Design review of the part built by this model. Coordinates are the model's own, in mm. A direction names the side the tool comes from. Give positions to 0.01 mm unless a question says otherwise; leave off trailing zeros. Loops run counter-clockwise (first coordinate to the right, second up) from the corner with the lowest first, then second, coordinate; pieces in that order, holes last. Notation, with made-up numbers: M 71.25,80.5 L 97.25,80.5 A14 cw 97.25,88.5 Z; hole C 52,87.25 d5. An arc over 180 degrees is marked long. Use a Markdown table: item, result. Add a question column.
(1) For probe 1 along Z at (x, y) = (63, 20); probe 2 along X at (y, z) = (20.5, 14); probe 3 along Z at (x, y) = (24, 15), list the stretches that pass through material, from the lowest coordinate up.
(2) Add section B-B, the plane x = -1.5. Give the boundary of the cut face in (y, z).
(3) Add section D-D, the plane x = 38.5. Give the boundary of the cut face in (y, z), then the cut area to 3 significant figures.
(4) Add section C-C, the plane z = 37. Give the boundary of the cut face in (x, y).
(5) Insertion check: pin 1 Ø24 at (x, y) = (53, 21) entering from -Z; pin 2 Ø15 at (x, z) = (2, 50) entering from -Y; pin 3 Ø12 at (x, y) = (11.5, 7.5) entering from -Z; pin 4 Ø5 at (x, y) = (-24, 26) entering from -Z. Each pin has a flat end and moves straight along its axis. Give the tip position at first contact, or say it passes through.
(6) Add section A-A, the plane z = 11. Give the boundary of the cut face in (x, y), then the cut area to 3 significant figures.
(7) Draft analysis for pull direction Z (two halves, no side actions). For faces 5 (the face through (23, 20, 18)), 6 (the face through (-50, 20, -15)), 7 (the face through (0, 7, -49)), state which applies: pulls with the +Z half, pulls with the -Z half, needs draft (parallel to the pull), parting line crosses it, or undercut.
(8) For faces 1 (the face through (18, 20, 23)), 2 (the face through (0, 33, 49)), 3 (the face through (-50, 20, 15)), 4 (the face through (49, 7, 0)), list the 3-axis set-ups (+Z, -Z, +X, -X, +Y, -Y) from which the entire face can be reached by the end or side of a thin tool; tool diameter is ignored.
```python
from build123d import *

# Parameters (mm, degrees)
CROQUIS1_W     = 40
CROQUIS1_H     = 50
CROQUIS1_H_2   = 40
CROQUIS1_W_2   = 50
EXTRUIR1_DEPTH = 40
CROQUIS2_W     = 40
CROQUIS2_H     = 40
CROQUIS2_W_2   = 30
CROQUIS2_H_2   = 30
EXTRUIR2_DEPTH = 40
CROQUIS3_W     = 40
CROQUIS3_H     = 40
CROQUIS3_W_2   = 30
CROQUIS3_H_2   = 30
EXTRUIR3_DEPTH = 40
CROQUIS5_W     = 40
CROQUIS5_H     = 40
CROQUIS5_W_2   = 30
CROQUIS5_H_2   = 30
EXTRUIR4_DEPTH = 40
CROQUIS6_W     = 40
CROQUIS6_H     = 40
CROQUIS6_W_2   = 30
CROQUIS6_H_2   = 30
EXTRUIR5_DEPTH = 40
VACIADO1_T     = -2


with BuildPart() as part:
    # Croquis1 → Extruir1 (new body)
    with BuildSketch(Plane(origin=(0, 0, 0), x_dir=(1, 0, 0), z_dir=(0, 1, 0))):
        with Locations((0, 45)):
            Rectangle(CROQUIS1_W, CROQUIS1_H)
        Rectangle(CROQUIS1_W, CROQUIS1_H_2)
        with Locations((45, 0)):
            Rectangle(CROQUIS1_W_2, CROQUIS1_H_2)
        with Locations((-45, 0)):
            Rectangle(CROQUIS1_W_2, CROQUIS1_H_2)
        with Locations((0, -45)):
            Rectangle(CROQUIS1_W, CROQUIS1_H)
    extrude(amount=EXTRUIR1_DEPTH)

    # Croquis2 → Extruir2 (cut)
    with BuildSketch(Plane(origin=(70, 0, 0), x_dir=(0, 0, -1), z_dir=(1, 0, 0))):
        with Locations((0, 20)):
            Rectangle(CROQUIS2_W, CROQUIS2_H)
        with Locations((0, 20)):
            Rectangle(CROQUIS2_W_2, CROQUIS2_H_2, mode=Mode.SUBTRACT)
    extrude(amount=-EXTRUIR2_DEPTH, mode=Mode.SUBTRACT)

    # Croquis3 → Extruir3 (cut)
    with BuildSketch(Plane(origin=(0, 0, -70), x_dir=(-1, 0, 0), z_dir=(0, 0, -1))):
        with Locations((0, 20)):
            Rectangle(CROQUIS3_W, CROQUIS3_H)
        with Locations((0, 20)):
            Rectangle(CROQUIS3_W_2, CROQUIS3_H_2, mode=Mode.SUBTRACT)
    extrude(amount=-EXTRUIR3_DEPTH, mode=Mode.SUBTRACT)

    # Croquis5 → Extruir4 (cut)
    with BuildSketch(Plane.ZY.offset(70)):
        with Locations((0, 20)):
            Rectangle(CROQUIS5_W, CROQUIS5_H)
        with Locations((0, 20)):
            Rectangle(CROQUIS5_W_2, CROQUIS5_H_2, mode=Mode.SUBTRACT)
    extrude(amount=-EXTRUIR4_DEPTH, mode=Mode.SUBTRACT)

    # Croquis6 → Extruir5 (cut)
    with BuildSketch(Plane.XY.offset(70)):
        with Locations((0, 20)):
            Rectangle(CROQUIS6_W, CROQUIS6_H)
        with Locations((0, 20)):
            Rectangle(CROQUIS6_W_2, CROQUIS6_H_2, mode=Mode.SUBTRACT)
    extrude(amount=-EXTRUIR5_DEPTH, mode=Mode.SUBTRACT)

    # Vaciado1
    vaciado1_openings = [part.faces().sort_by_distance(p)[0] for p in [
        (0, 20, 70),
        (70, 20, 0),
        (0, 20, -70),
        (-70, 20, 0),
    ]]
    offset(amount=VACIADO1_T, openings=vaciado1_openings, kind=Kind.INTERSECTION)


solid = part.part
```
Established:
| question | item | result |
|---|---|---|
| 1 | probe 1 | -15 to -13, 13 to 15 |
| 1 | probe 2 | -70 to -28, 28 to 70 |
| 1 | probe 3 | -20 to -18, 18 to 20 |
| 2 | outline | M 0,-30 L 5,-30 L 5,-70 L 7,-70 L 7,-28 L 2,-28 L 2,28 L 7,28 L 7,70 L 5,70 L 5,30 L 0,30 Z; M 33,-70 L 35,-70 L 35,-30 L 40,-30 L 40,30 L 35,30 L 35,70 L 33,70 L 33,28 L 38,28 L 38,-28 L 33,-28 Z |
| 3 | outline | M 5,-15 L 35,-15 L 35,15 L 5,15 Z; hole M 7,-13 L 33,-13 L 33,13 L 7,13 Z |
| 3 | area | 224 mm^2 |
| 4 | outline | M -15,5 L 15,5 L 15,35 L -15,35 Z; hole M -13,7 L 13,7 L 13,33 L -13,33 Z |
| 5 | pin 1 | z = -15 |
| 5 | pin 2 | y = 5 |
| 5 | pin 3 | z = -70 |
| 5 | pin 4 | z = -20 |
| 6 | outline | M -70,5 L -30,5 L -30,0 L 30,0 L 30,5 L 70,5 L 70,7 L 28,7 L 28,2 L -28,2 L -28,7 L -70,7 Z; M -70,33 L -28,33 L -28,38 L 28,38 L 28,33 L 70,33 L 70,35 L 30,35 L 30,40 L -30,40 L -30,35 L -70,35 Z |
| 6 | area | 600 mm^2 |
| 7 | face 5 | undercut |
| 7 | face 6 | pulls with the -Z half |
| 7 | face 7 | needs draft |
| 8 | face 1 | none |
| 8 | face 2 | +Z, -Z |
| 8 | face 3 | +Z, -X, +Y, -Y |
| 8 | face 4 | +X, -X |
